Geometry check sheet. Reference: the model listing, model coordinates, mm. Give positions to 0.01 mm unless a question says otherwise; leave off trailing zeros. Write each loop counter-clockwise with the first axis right and the second up, starting at its lowest first coordinate (ties: lowest second). Pieces come first, ordered by that corner, then holes. Notation, with made-up numbers: (46, 45.25) - (94, 45.25) arc R35 cw to (94, 81.25) - close; hole circle Ø10 at (44, 35.25). An arc over 180 degrees is marked (long way). One line per question, with ' | ' between items. Start each with the question number.
Q1. Thickness scan on L1, parallel to Z at x = 1, y = 34.1 (1 decimal); L2, parallel to Z at x = -4, y = 34.95 (1 decimal); L3, parallel to X at y = 34.9, z = 30. Record the ranges inside material, lowest first. Write a range as [from, to].
Q2. Section check A-A on x = -7. Record the boundary of the cut face in (y, z) (1 decimal).
Q3. Gauge pin test, flat ends, axial feed: P1, Ø4, axis at x = 1, z = -69.1, coming from the -Y side; P2, Ø1.5, axis at y = 34.5, z = -26, coming from the -X side; P3, Ø0.9, axis at x = -32, y = 34, coming from the -Z side. Record the tip position at first contact, or that the pin passes through.
Q4. Section check B-B on y = 34.4. Count the separate pieces of the cut face and the enclosed holes in it, and give its area (3 significant figures).
Q5. Section check C-C on z = -30.5. Record the boundary of the cut face in (x, y).
Autodesk Inventor part; units mm, degrees
ref_plane "YZ Plane" through (0, 0, 0) normal (1, 0, 0) x (0, 1, 0)
ref_plane "XZ Plane" through (0, 0, 0) normal (0, 1, 0) x (-1, 0, 0)
ref_plane "XY Plane" through (0, 0, 0) normal (0, 0, 1) x (1, 0, 0)
ref_plane "Work Plane1" through (-100.0042, 32.3083, -20.5972) normal (0, 1, 0) x (-1, 0, 0)
sketch "Sketch2" plane through (-100.0042, 32.3083, -20.5972) normal (0, 1, 0) x (-1, 0, 0)
  line L0 (-37.0577, 56.8227) -> (-118.6401, 56.8227)
  line L1 (-118.6401, 56.8227) -> (-118.6401, -55.8539)
  line L2 (-118.6401, -55.8539) -> (-95.0834, -55.8539)
  line L3 (-95.0834, -55.8539) -> (-95.0834, -41.3074)
  line L4 (-95.0834, -41.3074) -> (-106.1561, -41.3074)
  line L5 (-106.1561, -41.3074) -> (-106.1561, 43.3122)
  line L6 (-106.1561, 43.3122) -> (-91.4467, 43.3122)
  line L7 (-105, 46) -> (-105, -52.5)
  line L8 (-105, -52.5) -> (105, -52.5)
  line L9 (105, -52.5) -> (105, 52.5)
  line L10 (105, 52.5) -> (-93, 52.5)
  line L11 (-93, 52.5) -> (-93, 48)
  arc A0 (-95, 46) -> (-93, 48) centre (-95, 48) ccw
  line L12 (-95, 46) -> (-105, 46)
  circle A1 centre (-101, -48.5) radius 1.5
  circle A2 centre (101, -48.5) radius 2
  circle A3 centre (101, 27.5) radius 2
  circle A4 centre (-42.4, 49.5) radius 1.5
  circle A5 centre (-101, -48.5) radius 1.5
  circle A6 centre (-101, -48.5) radius 1.5
  circle A7 centre (-101, -48.5) radius 1.5
  circle A8 centre (-101, -48.5) radius 1.5
  circle A9 centre (-101, -48.5) radius 1.5
  circle A10 centre (-101, -48.5) radius 1.5
  circle A11 centre (-101, -48.5) radius 1.5
  circle A12 centre (-101, -48.5) radius 1.5
  circle A13 centre (-101, -48.5) radius 1.5
  circle A14 centre (-101, -48.5) radius 1.45
  circle A15 centre (-101, 49.5) radius 1.45
  line L13 (-91.4467, 50.0155) -> (-46.3722, 50.0155)
  line L14 (-46.3722, 50.0155) -> (-46.3722, 46)
  line L15 (-46.3722, 46) -> (-37.0577, 46)
  line L16 (-37.0577, 46) -> (-37.0577, 56.8227)
  line L17 (-91.4467, 43.3122) -> (-91.4467, 50.0155)
  circle A16 centre (-42.4, 49.5) radius 1.5
  point P0 (-100.0042, 20.5972)
  point P1 (-37.0577, 56.8227)
  dimension "d2" = 2.9
extrude "Extrusion1" add sketch "Sketch2" along normal blind 3 contours L16 L10 L11 A0 L12 L7 L6 L5 L4 L8 L3 L2 L1 L0 | L16 L15 L14 L13 L17 L6 L7 L12 A0 L11 L10 | L8 L7 L4 L3
properties part number "strut1"
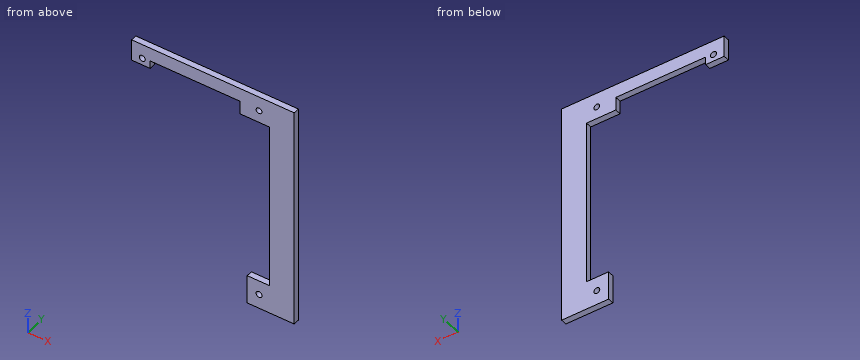
Working result:
1) L1: z = [-76.5, -70.6], [-67.6, -61.9], [22.7, 27.5], [30.4, 36.2] | L2: z = [-76.5, -61.9], [22.7, 36.2] | L3: x = [-62.95, -58.63], [-56.58, 0.05], [1.94, 18.64]
2) outline: (32.3, 22.7) - (35.3, 22.7) - (35.3, 36.2) - (32.3, 36.2) - close
3) P1: stops at y = 32.31 | P2: stops at x = 6.15 | P3: stops at z = 29.42
4) separate pieces: 1 | enclosed holes: 3 | area: 2,150 mm2
5) outline: (6.15, 32.31) - (18.64, 32.31) - (18.64, 35.31) - (6.15, 35.31) - close
